Job drawing, mm, ordinate dimensions from the low corner. One solid piece. Give positions to 0.01 mm unless a question says otherwise; leave off trailing zeros. Write each loop counter-clockwise with the first axis right and the second up, starting at its lowest first coordinate (ties: lowest second). Pieces come first, ordered by that corner, then holes. Notation, with made-up numbers: (82, -24.75) -> (87, -24.75) arc R31 ccw to (87, 6.25) -> close; hole circle Ø11 at (41.25, 52.25). An arc over 180 degrees is marked (long way). Put each result on its own line as item: value. Start each with the question number.
Item 1: Slice it at C-C, the plane y = 4.2. Give the number of separate pieces and of enclosed holes in the cut face, plus the area to 3 significant figures.
Item 2: Slice it at B-B, the plane z = 21.15. List the corners of the cut face in (x, y), plus the area to 3 significant figures.
Item 3: Two-plate mould, pull along X, no slides. Class the marked faces 1 and 2: pulls with the +X half, pulls with the -X half, needs draft (parallel to the pull), parting line crosses it, or undercut.
Item 4: Slice it at A-A, the plane x = 18. List the corners of the cut face in (y, z).
Item 5: Flat gauge pins, fed straight in: pin 1 Ø2.5 at (y, z) = (3, 2) entering from -X; pin 2 Ø2.5 at (x, y) = (3, 2.5) entering from +Z; pin 3 Ø2.5 at (x, y) = (9.5, 3.5) entering from +Z; pin 4 Ø1 at (x, z) = (22.5, 28.5) entering from -Y. Where does each tip first touch, or does it go through?
Item 6: Drill centre lines: line 1 along X through (y, z) = (3.1, 21.15); line 2 along Z through (x, y) = (68, 2.65); line 3 along X through (y, z) = (2.9, 40.5). Where is each one in solid material? Low to high.
Item 7: Slice it at D-D, the plane z = 44. List the corners of the cut face in (x, y), plus the area to 3 significant figures.
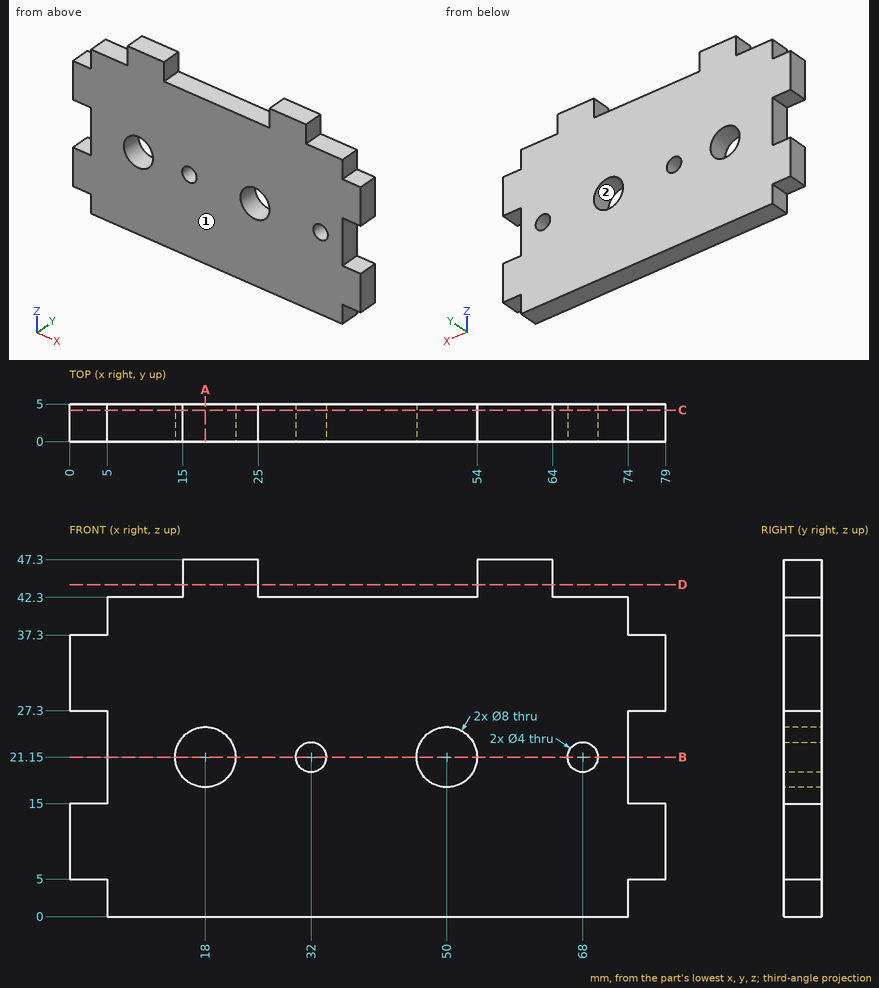
Values follow:
1. separate pieces: 1
1. enclosed holes: 4
1. area: 3,090 mm2
2. outline: (5, 0) -> (14, 0) -> (14, 5) -> (5, 5) -> close; (22, 0) -> (30, 0) -> (30, 5) -> (22, 5) -> close; (34, 0) -> (46, 0) -> (46, 5) -> (34, 5) -> close; (54, 0) -> (66, 0) -> (66, 5) -> (54, 5) -> close; (70, 0) -> (74, 0) -> (74, 5) -> (70, 5) -> close
2. area: 225 mm2
3. face 1: needs draft
3. face 2: undercut
4. outline: (0, 0) -> (5, 0) -> (5, 17.15) -> (0, 17.15) -> close; (0, 25.15) -> (5, 25.15) -> (5, 47.3) -> (0, 47.3) -> close
5. pin 1: x = 5
5. pin 2: z = 37.3
5. pin 3: z = 42.3
5. pin 4: y = 0
6. line 1: 5 to 14, 22 to 30, 34 to 46, 54 to 66, 70 to 74
6. line 2: 0 to 19.15, 23.15 to 42.3
6. line 3: 5 to 74
7. outline: (15, 0) -> (25, 0) -> (25, 5) -> (15, 5) -> close; (54, 0) -> (64, 0) -> (64, 5) -> (54, 5) -> close
7. area: 100 mm2
